Design review of the part built by this model. Coordinates are the model's own, in mm. Face numbers are marked on the shaded views. A direction names the side the tool comes from. Coordinates: 2 decimals unless noted, no trailing zeros. Order: outer loops, then holes, each group sorted by start corner. A loop starts at its lowest first (then second) coordinate and runs counter-clockwise, first axis right, second up. Notation, with made-up numbers: M 31,18.25 L 70,18.25 A14 ccw 70,37.25 Z; hole C 47.25,84 d1. An arc over 180 degrees is marked long. Answer as a JSON object with one key per item and string values.
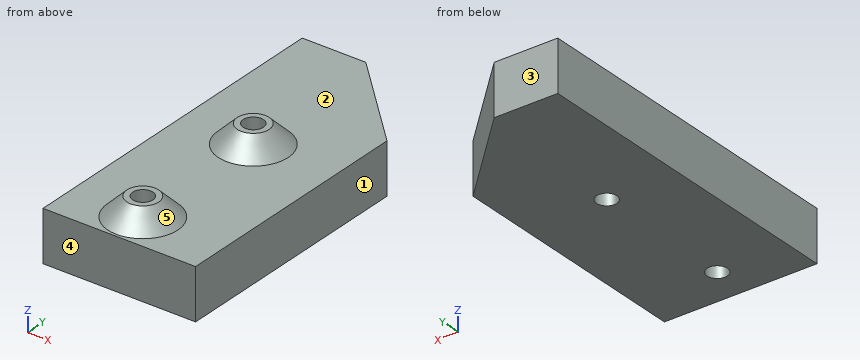
from build123d import *

# Parameters (mm, degrees)
CYLINDER082_R     = 0.8
CYLINDER082_DEPTH = 14.5
CYLINDER081_R     = 0.8
CYLINDER081_DEPTH = 14.5
BOX044_W          = 12
BOX044_H          = 26.75
BOX044_DEPTH      = 4
CHAMFER001_SIZE   = 7


with BuildPart() as cylinder134:
    # Cylinder082 → Cylinder082 (new body)
    with BuildSketch(Plane(origin=(-43.6, -13.8, -15), x_dir=(1, 0, 0), z_dir=(0, 0, 1))):
        Circle(CYLINDER082_R)
    extrude(amount=CYLINDER082_DEPTH)


with BuildPart() as fusion116:
    # Cylinder081 → Cylinder081 (new body)
    with BuildSketch(Plane(origin=(-43.6, -2.4, -15), x_dir=(1, 0, 0), z_dir=(0, 0, 1))):
        Circle(CYLINDER081_R)
    extrude(amount=CYLINDER081_DEPTH)

    # Fusion116: union Cylinder134
    add(cylinder134.part)


with BuildPart() as cone003:
    # Cone003 → Cone003 (revolve)
    with BuildSketch(Plane(origin=(-43.6, -13.8, -10), x_dir=(1, 0, 0), z_dir=(0, -1, 0))):
        Polygon((0, 0), (2.75, 0), (1.25, 1.5), (0, 1.5), align=None)
    revolve(axis=Axis((-43.6, -13.8, -10), (0, 0, 1)))


with BuildPart() as fusion114:
    # Cone002 → Cone002 (revolve)
    with BuildSketch(Plane(origin=(-43.6, -2.4, -10), x_dir=(1, 0, 0), z_dir=(0, -1, 0))):
        Polygon((0, 0), (2.75, 0), (1.25, 1.5), (0, 1.5), align=None)
    revolve(axis=Axis((-43.6, -2.4, -10), (0, 0, 1)))

    # Fusion114: union Cone003
    add(cone003.part)


with BuildPart() as cut045028:
    # Box044 → Box044 (new body)
    with BuildSketch(Plane(origin=(-50, -16.75, -14), x_dir=(1, 0, 0), z_dir=(0, 0, 1))):
        with Locations((6, 13.375)):
            Rectangle(BOX044_W, BOX044_H)
    extrude(amount=BOX044_DEPTH)

    # Chamfer001
    chamfer001_edges = [cut045028.edges().sort_by_distance(p)[0] for p in [
        (-50, 10, -12),
    ]]
    chamfer(chamfer001_edges, length=CHAMFER001_SIZE)

    # Fusion115: union Fusion114
    add(fusion114.part)

    # Cut045028: cut Fusion116
    add(fusion116.part, mode=Mode.SUBTRACT)


with BuildPart() as part_mirroring005:
    # Part__Mirroring005: instance of Cut045028
    add(cut045028.part.mirror(Plane(origin=(0, 0, 0), x_dir=(0, -1, 0), z_dir=(1, 0, 0))))


with BuildPart() as part_mirroring005_1:
    # Part__Mirroring005 placement: moved
    add(part_mirroring005.part.moved(Location((27, 0, 0))))


solid = part_mirroring005_1.part
1) Add section C-C (y = 2.5). State the section outline as (x, z) points, and give its area (3 significant figures).
Taken from the geometry:
{"outline": "M 65,-14 L 77,-14 L 77,-10 L 65,-10 Z", "area": "48.0 mm2"}
2) Add section A-A (x = 70.6). State the section outline as (y, z) points.
Taken from the geometry:
{"outline": "M -16.75,-14 L -14.6,-14 L -14.6,-8.5 L -15.05,-8.5 L -16.55,-10 L -16.75,-10 Z; M -13,-14 L -3.2,-14 L -3.2,-8.5 L -3.65,-8.5 L -5.15,-10 L -11.05,-10 L -12.55,-8.5 L -13,-8.5 Z; M -1.6,-14 L 9.4,-14 L 9.4,-10 L 0.35,-10 L -1.15,-8.5 L -1.6,-8.5 Z"}
3) Add section B-B (y = -2.4). State the section outline as (x, z) points.
Taken from the geometry:
{"outline": "M 65,-14 L 69.8,-14 L 69.8,-8.5 L 69.35,-8.5 L 67.85,-10 L 65,-10 Z; M 71.4,-14 L 77,-14 L 77,-10 L 73.35,-10 L 71.85,-8.5 L 71.4,-8.5 Z"}
4) Tool access review of the marked faces 1 and 2: name each direction out of +Z, -Z, +X, -X, +Y, -Y from which nothing blocks a thin tool from reaching the whole face with its end or side.
Taken from the geometry:
{"face 1": "+Z, -Z, +X, +Y, -Y", "face 2": "+Z"}
5) Insertion check: pin 1 Ø1.5 at (x, y) = (72, -8.5) entering from +Z; pin 2 Ø4 at (x, y) = (73.5, -12) entering from +Z; pin 3 Ø1.8 at (x, y) = (70.6, -13.8) entering from +Z; pin 4 Ø1.3 at (x, y) = (70.6, -2.4) entering from -Z. Each pin has a flat end and moves straight along its axis. Give the tip position at first contact, or say it passes through.
Taken from the geometry:
{"pin 1": "stops at z = -10", "pin 2": "stops at z = -8.66", "pin 3": "stops at z = -8.5", "pin 4": "passes through"}
6) To check wall thickness, follow L1, parallel to X at y = -2.4, z = -10.3; L2, parallel to Y at x = 70.6, z = -11; L3, parallel to Z at x = 68.75, y = -6.5. State the ranges of each line that lie inside material, in increasing order.
Taken from the geometry:
{"L1": "x = 65 to 69.8, 71.4 to 77", "L2": "y = -16.75 to -14.6, -13 to -3.2, -1.6 to 9.4", "L3": "z = -14 to -10"}
7) Mouldability with a two-part tool opening along Y and no side actions: class the marked faces 3, 4 and 5 as released by +Y, released by -Y, zero draft, split by the parting line, or undercut.
Taken from the geometry:
{"face 3": "released by +Y", "face 4": "released by -Y", "face 5": "undercut"}
8) Add section D-D (x = 66). State the section outline as (y, z) points.
Taken from the geometry:
{"outline": "M -16.75,-14 L 10,-14 L 10,-10 L -16.75,-10 Z"}
